```python
from build123d import *

# Parameters (mm, degrees)
SKETCH1_R           = 1.65
SKETCH1_R_2         = 1.642532795
BOSS_EXTRUDE1_DEPTH = 4.1


with BuildPart() as part:
    # Sketch1 → Boss-Extrude1 (new body)
    with BuildSketch(Plane.XY):
        Polygon((1, 2.483732861), (1, 42.483732861), (11, 42.483732861), (14, 22.483732861), (14, 2.483732861), align=None)
        with Locations((5, 6.483732861)):
            Circle(SKETCH1_R, mode=Mode.SUBTRACT)
        with Locations((5, 38.483732861)):
            Circle(SKETCH1_R_2, mode=Mode.SUBTRACT)
    extrude(amount=BOSS_EXTRUDE1_DEPTH)


solid = part.part
```
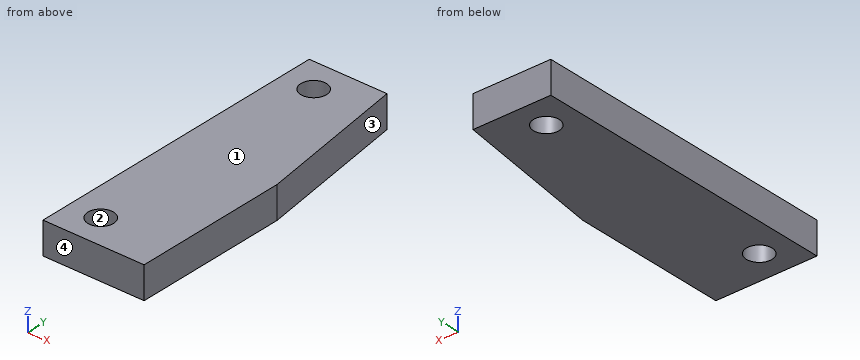
Work out the finished part from the listing and answer in its coordinate system (mm). Face numbers are marked on the shaded views. Give positions to 0.01 mm unless a question says otherwise; leave off trailing zeros. Loops run counter-clockwise (first coordinate to the right, second up) from the corner with the lowest first, then second, coordinate; pieces in that order, holes last. Notation, with made-up numbers: (12.25, 46) -> (43.25, 46) arc R17 cw to (43.25, 76) -> close; hole circle Ø2 at (2.5, 24.5). An arc over 180 degrees is marked (long way). Write item = value, one per line. Start each with the question number.
(1) Find section B-B on z = 3.15. Give the vertices of the cut face in (x, y).
(2) Find the intervals of material crossed by probe 1 along Y at (x, z) = (5, 1.6); probe 2 along X at (y, z) = (6.5, 3); probe 3 along X at (y, z) = (7.5, 2.25), in increasing order. Write a range as from..to.
(3) Find section D-D on x = 12.5. Give the vertices of the cut face in (y, z).
(4) Find section C-C on y = 34. Give the vertices of the cut face in (x, z).
(5) The mould has two halves that part along Y. Classify the marked faces 1, 2, 3 and 4: +Y half, -Y half, draft (parallel to the pull), parting line (faces both ways), or undercut.
(6) Find section A-A on x = 5. Give the vertices of the cut face in (y, z).
From the geometry:
q1.outline = (1, 2.48) -> (14, 2.48) -> (14, 22.48) -> (11, 42.48) -> (1, 42.48) -> close; hole circle Ø3.3 at (5, 6.48); hole circle Ø3.29 at (5, 38.48)
q2.probe_1 = 2.48..4.83, 8.13..36.84, 40.13..42.48
q2.probe_2 = 1..3.35, 6.65..14
q2.probe_3 = 1..3.7, 6.3..14
q3.outline = (2.48, 0) -> (32.48, 0) -> (32.48, 4.1) -> (2.48, 4.1) -> close
q4.outline = (1, 0) -> (12.27, 0) -> (12.27, 4.1) -> (1, 4.1) -> close
q5.face_1 = draft
q5.face_2 = undercut
q5.face_3 = +Y half
q5.face_4 = -Y half
q6.outline = (2.48, 0) -> (4.83, 0) -> (4.83, 4.1) -> (2.48, 4.1) -> close; (8.13, 0) -> (36.84, 0) -> (36.84, 4.1) -> (8.13, 4.1) -> close; (40.13, 0) -> (42.48, 0) -> (42.48, 4.1) -> (40.13, 4.1) -> close
